from build123d import *

# Parameters (mm, degrees)
BOSS_EXTRUDE1_DEPTH = 0.79375
SKETCH3_R           = 7.9375
BOSS_EXTRUDE2_DEPTH = 1.5875
BOSS_EXTRUDE3_DEPTH = 1.1176
SKETCH5_R           = 3.7830125
BOSS_EXTRUDE4_DEPTH = 0.5588
SKETCH7_R           = 1.905
BOSS_EXTRUDE5_DEPTH = 1.5875


with BuildPart() as part:
    # Sketch2 → Boss-Extrude1 (new body)
    with BuildSketch(Plane.XY):
        with BuildLine():
            Line((-10.570159202, -14.977509548), (0, -7.9375))
            ThreePointArc((0, -7.9375), (5.612660076, 5.612660076), (-7.9375, 0))
            Line((-7.9375, 0), (-14.977509548, -10.570159202))
            ThreePointArc((-14.977509548, -10.570159202), (-16.449796179, -11.80639255), (-17.00096249, -13.64816249))
            Line((-17.00096249, -13.64816249), (-21.49109055, -18.13829055))
            Line((-21.49109055, -18.13829055), (-18.13829055, -21.49109055))
            Line((-18.13829055, -21.49109055), (-13.64816249, -17.00096249))
            ThreePointArc((-13.64816249, -17.00096249), (-11.80639255, -16.449796179), (-10.570159202, -14.977509548))
        make_face()
    extrude(amount=BOSS_EXTRUDE1_DEPTH)

    # Sketch3 → Boss-Extrude2 (add)
    with BuildSketch(Plane.XY.offset(0.79375)):
        with Locations(Location((0, 0, 0), (0, 0, 180))):
            Circle(SKETCH3_R)
    extrude(amount=BOSS_EXTRUDE2_DEPTH)

    # Sketch4 → Boss-Extrude3 (add)
    with BuildSketch(Plane.XY.offset(2.38125)):
        Polygon((-5.349987584, 0), (0, -5.349987584), (13.027765396, 7.677777811), (10.352771604, 10.352771604), (21.444773795, 21.444773795), (20.283005592, 22.617844825), (15.977877039, 18.354197239), (15.63941792, 18.695949223), (19.937213299, 22.952334291), (18.769780003, 24.119767587), align=None)
    extrude(amount=BOSS_EXTRUDE3_DEPTH)

    # Sketch5 → Boss-Extrude4 (add)
    with BuildSketch(Plane.XY.offset(3.49885)):
        with Locations(Location((0, 0, 0), (0, 0, 225))):
            Circle(SKETCH5_R)
    extrude(amount=BOSS_EXTRUDE4_DEPTH)

    # Sketch7 → Boss-Extrude5 (add)
    with BuildSketch(Plane(origin=(0, 0, 0), x_dir=(-1, 0, 0), z_dir=(0, 0, -1))):
        with Locations(Location((0, 0, 0), (0, 0, 180))):
            Circle(SKETCH7_R)
    extrude(amount=BOSS_EXTRUDE5_DEPTH)


solid = part.part
Check sheet for the modelled part. Datum: model origin and axes. Units: mm. A direction names the side the tool comes from. Round coordinates to 2 decimals unless told otherwise and drop trailing zeros. Loops run counter-clockwise (first coordinate to the right, second up) from the corner with the lowest first, then second, coordinate; pieces in that order, holes last. Notation, with made-up numbers: (9, -5) -> (43, -5) arc R32 ccw to (43, 28) -> close; hole circle Ø3 at (-7, 60.5). An arc over 180 degrees is marked (long way). Put each result on its own line as item: value. Start each with the question number.
1. Section check B-B (y = -9.5). Enter the section's corners in (x, z).
2. Draft check along Y on faces 1 (the face through (-2.71, -2.64, 2.93)), 2 (the face through (-4, 0, 3.499)), 3 (the face through (18.161, 20.516, 2.932)), 4 (the face through (-19.21, -15.86, 0.39)). Enter one of: +Y half, -Y half, draft (parallel to the pull), parting line (faces both ways), or undercut.
3. Gauge pin test, flat ends, axial feed: pin 1 (23.5 mm diameter, centred on x = 0.5, y = -6, fed in from -Z); pin 2 (1.3 mm diameter, centred on x = -0.5, y = -4.5, fed in from +Z); pin 3 (1 mm diameter, centred on x = -12, y = -4.5, fed in from +Z); pin 4 (10.5 mm diameter, centred on x = -7, y = -9, fed in from +Z). Record the tip position at first contact, or that the pin passes through.
4. Scan lines: probe 1 along Z at (x, y) = (-16.5, -17.5); probe 2 along Z at (x, y) = (8, 7.5); probe 3 along Y at (x, z) = (-20, 0.7). Record each from-to range of solid material in increasing order.
5. Section check C-C (x = -10). Enter the section's corners in (y, z).
6. Access from +Z, -Z, +X, -X, +Y, -Y to the whole of each face (thin tool, end or side, straight path). Record for faces 5 (the face through (0.818, -3.694, 3.774)), 6 (the face through (11.709, 8.997, 2.932)), 7 (the face through (-12, -11, 0.794)).
7. Section check A-A (x = 11.5). Enter the section's corners in (y, z), plus the area to 3 significant figures.
Findings:
1. outline: (-14.26, 0) -> (-2.35, 0) -> (-2.35, 0.79) -> (-14.26, 0.79) -> close
2. face 1: -Y half
2. face 2: draft
2. face 3: undercut
2. face 4: +Y half
3. pin 1: stops at z = -1.59
3. pin 2: stops at z = 3.5
3. pin 3: passes through
3. pin 4: stops at z = 2.38
4. probe 1: z = 0 to 0.79
4. probe 2: z = 2.38 to 3.5
4. probe 3: y = -19.63 to -16.65
5. outline: (-14.6, 0) -> (-3.1, 0) -> (-3.1, 0.79) -> (-14.6, 0.79) -> close
6. face 5: +Z
6. face 6: +Z, -Z, +X
6. face 7: +Z, -X, -Y
7. outline: (6.15, 2.38) -> (9.21, 2.38) -> (9.21, 3.5) -> (6.15, 3.5) -> close; (11.5, 2.38) -> (16.85, 2.38) -> (16.85, 3.5) -> (11.5, 3.5) -> close
7. area: 9.39 mm^2
